The model under review builds one solid part; all positions refer to its coordinate system, in mm. Face numbers are marked on the shaded views. Round coordinates to 2 decimals unless told otherwise and drop trailing zeros. Write each loop counter-clockwise with the first axis right and the second up, starting at its lowest first coordinate (ties: lowest second). Pieces come first, ordered by that corner, then holes. Notation, with made-up numbers: (-8, 65.25) -> (3, 65.25) arc R20 ccw to (3, 79.25) -> close; hole circle Ø3 at (29, 78.5). An arc over 180 degrees is marked (long way). Answer as a JSON object with one key per item and string values. Group by question number.
1) Insertion check: pin 1 Ø1 at (y, z) = (0.5, -61.5) entering from +X; pin 2 Ø1 at (y, z) = (-3, -36) entering from +X; pin 3 Ø5.5 at (x, y) = (0, 0) entering from +Z; pin 4 Ø5 at (x, z) = (-9, -30) entering from -Y. Each pin has a flat end and moves straight along its axis. Give the tip position at first contact, or say it passes through.
2) We need section D-D, the plane z = -21. Write out the cut boundary in (x, y).
3) Mouldability with a two-part tool opening along X and no side actions: class the marked faces 1, 2, 3 and 4 as pulls with the +X half, pulls with the -X half, needs draft (parallel to the pull), parting line crosses it, or undercut.
4) To check wall thickness, follow probe 1 along Y at (x, z) = (0, -18.5); probe 2 along Y at (x, z) = (0, -49.5); probe 3 along X at (y, z) = (-0.25, -63.5). State the ranges of each line that lie inside material, in increasing order. Write a range as [from, to].
5) We need section A-A, the plane x = 0. Write out the cut boundary in (y, z).
6) We need section C-C, the plane z = -53. Write out the cut boundary in (x, y), then the cut area to 3 significant figures.
Solid Edge part; units mm, degrees
sketch "Sketch1" plane through (0, 0, 0) normal (0, 0, 1) x (1, 0, 0)
  circle A0 centre (0, 0) radius 15
extrude "Extrusionsausprägung_22" add sketch "Sketch1" against normal blind 5
sketch "Sketch2" plane through (0, 0, -5) normal (0, 0, -1) x (1, 0, 0)
  circle A0 centre (0, 0) radius 9
extrude "Extrusionsausprägung_23" add sketch "Sketch2" along normal blind 70
sketch "Sketch3" plane through (0, 0, -75) normal (0, 0, -1) x (1, 0, 0)
  circle A0 centre (0, 0) radius 4.65
extrude "Extrusionsausschnitt_30" cut sketch "Sketch3" against normal blind 89
sketch "Sketch4" plane through (0, 0, 0) normal (0, 0, 1) x (-1, 0, 0)
  circle A0 centre (0, 0) radius 7
extrude "Extrusionsausschnitt_31" cut sketch "Sketch4" against normal blind 30
chamfer "Fase_11" distance 3 angle 45 1 edges at (7, 0, -30)
chamfer "Fase_12" distance 0.5 angle 45 2 edges at (7, 0, 0) (-15, 0, 0)
chamfer "Fase_13" distance 2 angle 45 1 edges at (-9, 0, -5)
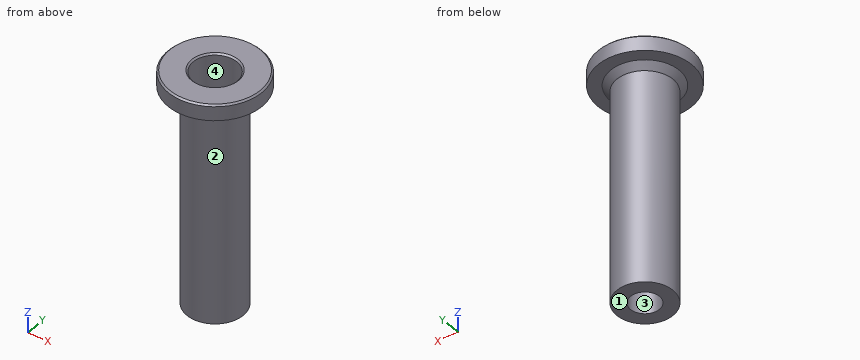
Here are the results:
{
 "1": {"pin 1": "stops at x = 9", "pin 2": "stops at x = 8.65", "pin 3": "passes through", "pin 4": "stops at y = -6.22"},
 "2": {"outline": "circle Ø18 at (0, 0); hole circle Ø14 at (0, 0)"},
 "3": {"face 1": "needs draft", "face 2": "parting line crosses it", "face 3": "undercut", "face 4": "undercut"},
 "4": {"probe 1": "y = [-9, -7], [7, 9]", "probe 2": "y = [-9, -4.65], [4.65, 9]", "probe 3": "x = [-9, -4.64], [4.64, 9]"},
 "5": {"outline": "(-15, -5) -> (-11, -5) -> (-9, -7) -> (-9, -75) -> (-4.65, -75) -> (-4.65, -29.35) -> (-7, -27) -> (-7, -0.5) -> (-7.5, 0) -> (-14.5, 0) -> (-15, -0.5) -> close; (4.65, -75) -> (9, -75) -> (9, -7) -> (11, -5) -> (15, -5) -> (15, -0.5) -> (14.5, 0) -> (7.5, 0) -> (7, -0.5) -> (7, -27) -> (4.65, -29.35) -> close"},
 "6": {"outline": "circle Ø18 at (0, 0); hole circle Ø9.3 at (0, 0)", "area": "187 mm^2"}
}
